Could you check a few things on this model? Use its own coordinates, in mm. Face numbers are marked on the shaded views. A direction names the side the tool comes from. Give positions to 0.01 mm unless a question says otherwise; leave off trailing zeros. Write each loop counter-clockwise with the first axis right and the second up, starting at its lowest first coordinate (ties: lowest second). Pieces come first, ordered by that corner, then holes. Notation, with made-up numbers: (67.25, 23) - (125.25, 23) arc R18 ccw to (125.25, 52) - close; hole circle Ø8 at (32, 39). An arc over 180 degrees is marked (long way). Answer in a Markdown table with one row per item.
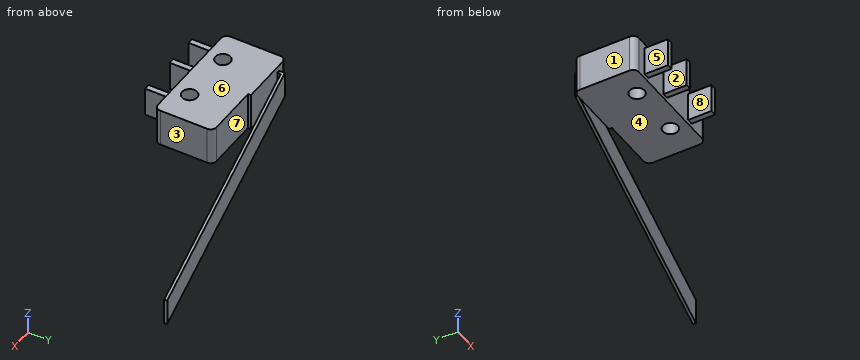
from build123d import *

# Parameters (mm, degrees)
BOSS_EXTRUDE1_DEPTH  = 6.5
FILLET1_R            = 1
M2_CLEARANCE_HOLE1_D = 2.6
BOSS_EXTRUDE2_START  = -1
BOSS_EXTRUDE2_DEPTH  = 4.5
SKETCH6_W            = 1
SKETCH6_H            = 5
BOSS_EXTRUDE3_DEPTH  = 4


with BuildPart() as part:
    # Sketch1 → Boss-Extrude1 (new body)
    with BuildSketch(Plane.XY):
        Polygon((10, 10.6), (10, 10.1), (20, 10.1), (20, 0), (0, 0), (0, 10.6), align=None)
    extrude(amount=BOSS_EXTRUDE1_DEPTH)

    # Fillet1
    fillet1_edges = [part.edges().sort_by_distance(p)[0] for p in [
        (0, 10.6, 3.25),
        (20, 10.1, 3.25),
        (20, 0, 3.25),
        (0, 0, 3.25),
    ]]
    fillet(fillet1_edges, radius=FILLET1_R)

    # M2 Clearance Hole1 (through all)
    with Locations(Plane.XY.offset(6.5)):
        with Locations((5.1, 2.8), (14.6, 2.8)):
            Hole(M2_CLEARANCE_HOLE1_D / 2)

    # Sketch5 → Boss-Extrude2 (add)
    with BuildSketch(Plane.XY.offset(6.5).offset(BOSS_EXTRUDE2_START)):
        Polygon((2, 11.6), (2, 10.6), (2.5, 10.6), (2.5, 11.201813956), (56.104500003, 23.512686364), (55.992582981, 24), align=None)
    extrude(amount=-BOSS_EXTRUDE2_DEPTH)

    # Sketch6 → Boss-Extrude3 (add)
    with BuildSketch(Plane.XZ):
        with Locations((3.159009098, 3.25)):
            Rectangle(SKETCH6_W, SKETCH6_H)
        with Locations((8.531370471, 3.25)):
            Rectangle(SKETCH6_W, SKETCH6_H)
        with Locations((15.53592061, 3.25)):
            Rectangle(SKETCH6_W, SKETCH6_H)
    extrude(amount=BOSS_EXTRUDE3_DEPTH)


solid = part.part
1) Imagine slicing it at D-D (y = 6.5). List the corners of the cut face in (x, z) for me.
Check values:
| item | result |
|---|---|
| outline | (0, 0) - (20, 0) - (20, 6.5) - (0, 6.5) - close |
2) We'd pull the mould along X, two halves only. Please class the marked faces 1, 2 and 3: +X half, -X half, draft (parallel to the pull), parting line (faces both ways), or undercut.
Check values:
| item | result |
|---|---|
| face 1 | -X half |
| face 2 | undercut |
| face 3 | +X half |
3) If I drill on line 1 (Y direction, x = 14.6, z = 2.5); line 2 (Y direction, x = 5.1, z = 3.5); line 3 (Z direction, x = 8, y = 12.5), over which ranges is the centre line in solid material (lowest first)?
Check values:
| item | result |
|---|---|
| line 1 | y = 0 to 1.5, 4.1 to 10.1, 13.98 to 14.49 |
| line 2 | y = 0 to 1.5, 4.1 to 10.6, 11.8 to 12.31 |
| line 3 | z = 1 to 5.5 |
4) Will these pins go through, and if not, where does the flat tip stop? P1, Ø3, axis at x = 45.5, z = 2.5, coming from the -Y side; P2, Ø2, axis at x = 31, z = 2, coming from the +Y side; P3, Ø6.5, axis at x = 24, y = 17, coming from the -Z side.
Check values:
| item | result |
|---|---|
| P1 | stops at y = 20.73 |
| P2 | stops at y = 18.49 |
| P3 | stops at z = 1 |
5) Imagine slicing it at B-B (y = 2.8). List the corners of the cut face in (x, z) for me.
Check values:
| item | result |
|---|---|
| outline | (0, 0) - (3.8, 0) - (3.8, 6.5) - (0, 6.5) - close; (6.4, 0) - (13.3, 0) - (13.3, 6.5) - (6.4, 6.5) - close; (15.9, 0) - (20, 0) - (20, 6.5) - (15.9, 6.5) - close |
6) On a 3-axis mill with a long thin cutter (end or side, diameter ignored), from which of +Z, -Z, +X, -X, +Y, -Y can I reach the whole of each face in a straight line? I mean the marked faces 4, 5, 6, 7 and 8. Say none if no direction works.
Check values:
| item | result |
|---|---|
| face 4 | -Z, +X, -X, +Y, -Y |
| face 5 | +Z, -Z, -X, -Y |
| face 6 | +Z, +X, -X, +Y, -Y |
| face 7 | +Z, -Z, +X |
| face 8 | +Z, -Z, -Y |
7) Imagine slicing it at C-C (x = 5.1). List the corners of the cut face in (y, z) for me.
Check values:
| item | result |
|---|---|
| outline | (0, 0) - (1.5, 0) - (1.5, 6.5) - (0, 6.5) - close; (4.1, 0) - (10.6, 0) - (10.6, 6.5) - (4.1, 6.5) - close; (11.8, 1) - (12.31, 1) - (12.31, 5.5) - (11.8, 5.5) - close |
8) Imagine slicing it at A-A (z = 2.5). State how many separate pieces and enclosed holes the cut face has, then the cut area to 3 significant figures.
Check values:
| item | result |
|---|---|
| separate pieces | 1 |
| enclosed holes | 2 |
| area | 236 mm2 |
